Source: CAD feature listing. Evaluate the final solid. Frame: model axes, mm. Face numbers are marked on the shaded views. A direction names the side the tool comes from. Give positions to 0.01 mm unless a question says otherwise; leave off trailing zeros. Loops run counter-clockwise (first coordinate to the right, second up) from the corner with the lowest first, then second, coordinate; pieces in that order, holes last. Notation, with made-up numbers: M 30.5,69.5 L 37.5,69.5 A32 cw 37.5,100.5 Z; hole C 17.5,47 d11. An arc over 180 degrees is marked long. Put each result on its own line as item: value.
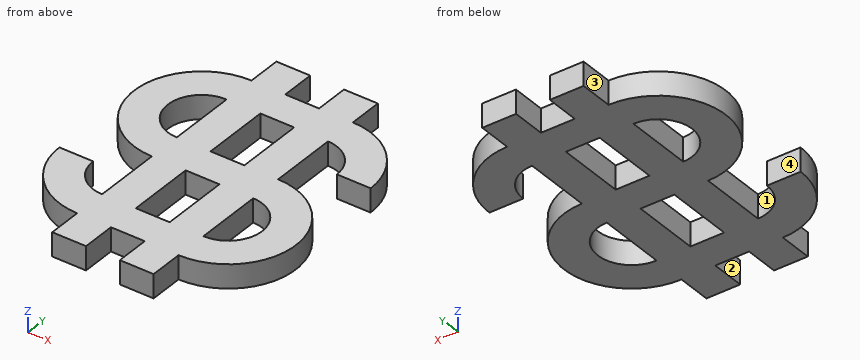
from build123d import *

# Parameters (mm, degrees)
F0_W     = 4.2857142857
F0_H     = 4.2857142857
F0_H_2   = 8.5714285714
F1_DEPTH = 3
F2_DEPTH = 3


with BuildPart() as f1:
    # F0 (on Top) → F1 (new body)
    with BuildSketch(Plane.XY):
        with BuildLine():
            ThreePointArc((-8.5714285714, 4.2857142857), (-5.5409709378, 3.0304576337), (-4.2857142857, 0))
            Line((-4.2857142857, 0), (0, 0))
            ThreePointArc((0, 0), (-2.5105133041, 6.0609152673), (-8.5714285714, 8.5714285714))
            Line((-8.5714285714, 8.5714285714), (-8.5714285714, 4.2857142857))
        make_face()
        with Locations((-10.7142857143, 6.4285714286)):
            Rectangle(F0_W, F0_H)
        with Locations((-10.7142857143, 10.7142857143)):
            Rectangle(F0_W, F0_H)
        with Locations((-15, 6.4285714286)):
            Rectangle(F0_W, F0_H)
        with Locations((-10.7142857143, 0)):
            Rectangle(F0_W, F0_H_2)
        Polygon((-17.1428571429, 0), (-17.1428571429, 4.2857142857), (-21.4285714286, 4.2857142857), (-21.4285714286, -4.2857142857), (-17.1428571429, -4.2857142857), align=None)
        with Locations((-19.2857142857, 6.4285714286)):
            Rectangle(F0_W, F0_H)
        with Locations((-19.2857142857, 10.7142857143)):
            Rectangle(F0_W, F0_H)
    extrude(amount=F1_DEPTH)

    # F0 (on Top) → F2 (join)
    with BuildSketch(Plane.XY):
        with BuildLine():
            ThreePointArc((-21.4285714286, -4.2857142857), (-25.7142857143, 0), (-21.4285714286, 4.2857142857))
            Line((-21.4285714286, 4.2857142857), (-21.4285714286, 8.5714285714))
            ThreePointArc((-21.4285714286, 8.5714285714), (-30, 0), (-21.4285714286, -8.5714285714))
            Line((-21.4285714286, -8.5714285714), (-21.4285714286, -4.2857142857))
        make_face()
        with Locations((-19.2857142857, -6.4285714286)):
            Rectangle(F0_W, F0_H)
        with Locations((-19.2857142857, -12.8571428571)):
            Rectangle(F0_W, F0_H_2)
        with BuildLine():
            ThreePointArc((-8.5714285714, -21.4285714286), (0, -12.8571428571), (-8.5714285714, -4.2857142857))
            Line((-8.5714285714, -4.2857142857), (-8.5714285714, -8.5714285714))
            ThreePointArc((-8.5714285714, -8.5714285714), (-4.2857142857, -12.8571428571), (-8.5714285714, -17.1428571429))
            Line((-8.5714285714, -17.1428571429), (-8.5714285714, -21.4285714286))
        make_face()
        with Locations((-10.7142857143, -19.2857142857)):
            Rectangle(F0_W, F0_H)
        with Locations((-15, -19.2857142857)):
            Rectangle(F0_W, F0_H)
        with Locations((-19.2857142857, -19.2857142857)):
            Rectangle(F0_W, F0_H)
        with Locations((-10.7142857143, -6.4285714286)):
            Rectangle(F0_W, F0_H)
        with BuildLine():
            ThreePointArc((-30, -12.8571428571), (-27.4894866959, -18.9180581245), (-21.4285714286, -21.4285714286))
            Line((-21.4285714286, -21.4285714286), (-21.4285714286, -17.1428571429))
            ThreePointArc((-21.4285714286, -17.1428571429), (-24.4590290622, -15.8876004908), (-25.7142857143, -12.8571428571))
            Line((-25.7142857143, -12.8571428571), (-30, -12.8571428571))
        make_face()
        with Locations((-19.2857142857, -23.5714285714)):
            Rectangle(F0_W, F0_H)
        with Locations((-10.7142857143, -23.5714285714)):
            Rectangle(F0_W, F0_H)
        with Locations((-10.7142857143, -12.8571428571)):
            Rectangle(F0_W, F0_H_2)
        with Locations((-15, -6.4285714286)):
            Rectangle(F0_W, F0_H)
    extrude(amount=F2_DEPTH)


solid = f1.part
1. Access query for the marked faces 1, 2, 3 and 4. Directions: +Z, -Z, +X, -X, +Y, -Y. A direction counts if a zero-diameter tool reaches every point of the face in a straight line with its end or side. Return the directions, or none.
Found:
face 1: +Z, -Z
face 2: +Z, -Z, -Y
face 3: +Z, -Z, -X, +Y
face 4: +Z, -Z, -X
2. Contact query for flat-ended pins moving along their axis: P1, Ø5, axis at x = -14.5, y = -1, coming from the +Z side; P2, Ø1.5, axis at y = 4.5, z = 1.5, coming from the -X side; P3, Ø0.9, axis at y = 1, z = 1.5, coming from the -X side; P4, Ø1.5, axis at y = 10, z = 2, coming from the -X side. Output: stop coordinate, or through.
Found:
P1: z = 3
P2: x = -29.14
P3: x = -29.98
P4: x = -21.43
3. Section query D-D (y = -3.5). Output: boundary loops of the cut face in (x, z).
Found:
outline: M -29.25,0 L -23.9,0 L -23.9,3 L -29.25,3 Z; M -21.43,0 L -17.14,0 L -17.14,3 L -21.43,3 Z; M -12.86,0 L -8.57,0 L -8.57,3 L -12.86,3 Z
4. Material intervals for line 1 (Y direction, x = -14.25, z = 2.6); line 2 (X direction, y = -3.5, z = 2.6); line 3 (X direction, y = -22, z = 0.9), sorted ascending. Write a range as from..to.
Found:
line 1: -21.43..-17.14, -8.57..-4.29, 4.29..8.57
line 2: -29.25..-23.9, -21.43..-17.14, -12.86..-8.57
line 3: -21.43..-17.14, -12.86..-8.57
5. Section query A-A (y = -14). Output: boundary loops of the cut face in (x, z), plus the area to 3 significant figures.
Found:
outline: M -29.92,0 L -25.56,0 L -25.56,3 L -29.92,3 Z; M -21.43,0 L -17.14,0 L -17.14,3 L -21.43,3 Z; M -12.86,0 L -8.57,0 L -8.57,3 L -12.86,3 Z; M -4.44,0 L -0.08,0 L -0.08,3 L -4.44,3 Z
area: 51.9 mm^2
6. Section query C-C (z = 1). State how many separate pieces and enclosed holes the cut face has, plus the area to 3 significant figures.
Found:
separate pieces: 1
enclosed holes: 4
area: 645 mm^2
7. Section query B-B (y = -9.5). Output: boundary loops of the cut face in (x, z), plus the area to 3 significant figures.
Found:
outline: M -21.43,0 L -17.14,0 L -17.14,3 L -21.43,3 Z; M -12.86,0 L -8.57,0 L -8.57,3 L -12.86,3 Z; M -5.91,0 L -0.68,0 L -0.68,3 L -5.91,3 Z
area: 41.4 mm^2
